Part print with two shaded views. Sizes in mm from the minimum x, y, z corner. A direction names the side the tool comes from. Coordinates: 2 decimals unless noted, no trailing zeros. Loops run counter-clockwise (first coordinate to the right, second up) from the corner with the lowest first, then second, coordinate; pieces in that order, holes last. Notation, with made-up numbers: (-34.5, -29) - (-0.5, -29) arc R22 ccw to (-0.5, 1) - close; hole circle Ø5 at (-4, 29.5). An arc over 180 degrees is marked (long way). Write each question's results on one line, items separated by ' | '. Start each with the question number.
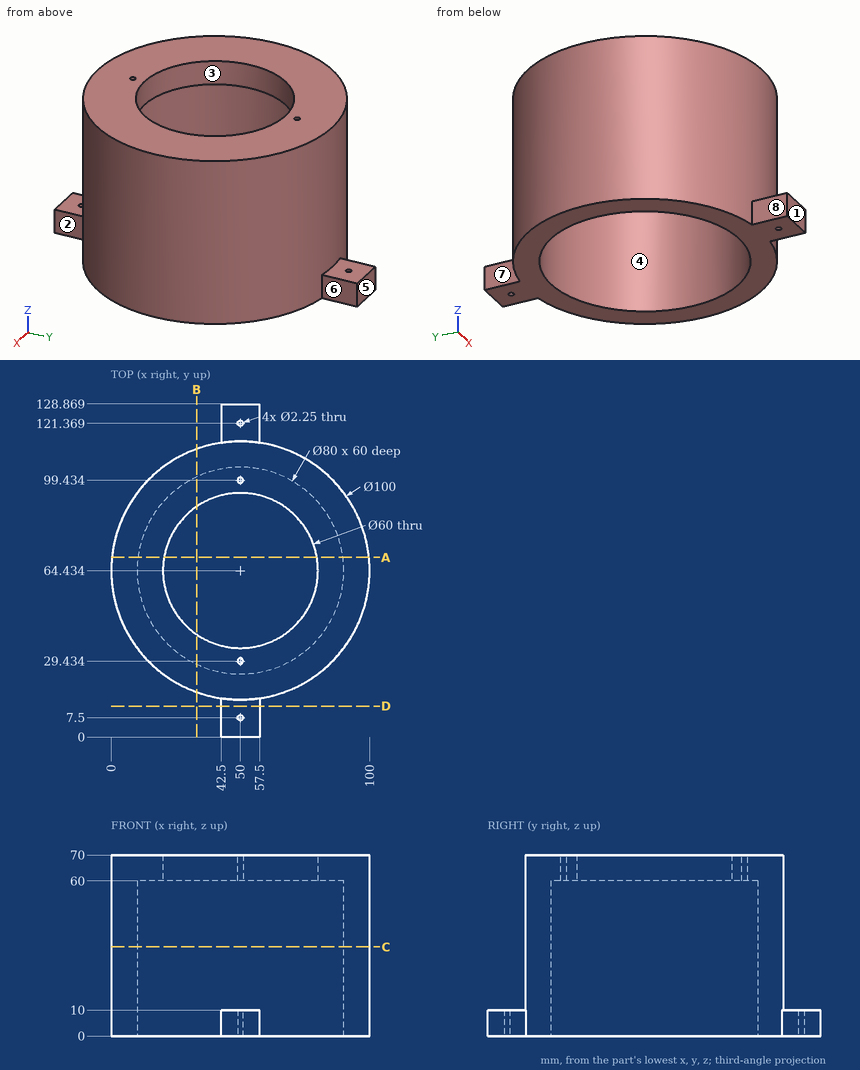
Q1. Pin check, flat tips, straight feed: pin 1 (12 mm diameter, centred on y = 53, z = 58.5, fed in from +X); pin 2 (4.5 mm diameter, centred on x = 53, y = 122.5, fed in from +Z); pin 3 (10 mm diameter, centred on x = 68, z = 17, fed in from +Y) (1 decimal). Stop position of each tip, or through.
Q2. Mould opens along Y. For the marked faces 1, 2 and 3 say: +Y half, -Y half, draft (parallel to the pull), parting line (faces both ways), or undercut.
Q3. Cut at A-A (y = 69.5). List the corners of the cut face in (x, z), and give its area (3 significant figures).
Q4. Cut at D-D (y = 12). List the corners of the cut face in (x, z), and give its area (3 significant figures).
Q5. Drill centre lines: L1, parallel to Y at x = 50, z = 62.5 (1 decimal); L2, parallel to Y at x = 48.5, z = 58; L3, parallel to Y at x = 50, z = 3.5 (1 decimal). Where is each one in solid material? Low to high. Write a range as from..to.
Q6. Which spindle directions (+Z, -Z, +X, -X, +Y, -Y) get a long thin tool onto all of the face, cutting with end or side? Do the marked faces 4, 5, 6, 7 and 8. Say none if no direction does.
Q7. Cut at C-C (z = 34.5). List the corners of the cut face in (x, y) (1 decimal), and give its area (3 significant figures).
Q8. Cut at B-B (x = 33). List the corners of the cut face in (y, z) (1 decimal).
Check result:
1) pin 1: x = 99.7 | pin 2: z = 10 | pin 3: y = 112.7
2) face 1: -Y half | face 2: draft | face 3: undercut
3) outline: (0.26, 0) - (10.32, 0) - (10.32, 60) - (20.43, 60) - (20.43, 70) - (0.26, 70) - close; (79.57, 60) - (89.68, 60) - (89.68, 0) - (99.74, 0) - (99.74, 70) - (79.57, 70) - close | area: 1,610 mm²
4) outline: (42.5, 0) - (57.5, 0) - (57.5, 10) - (42.5, 10) - close | area: 150 mm²
5) L1: 14.4..28.3, 30.6..34.4, 94.4..98.3, 100.6..114.4 | L2: 14.46..24.46, 104.41..114.41 | L3: 0..6.4, 8.6..24.4, 104.4..120.2, 122.5..128.9
6) face 4: -Z | face 5: +Z, -Z, +X, -X, +Y | face 6: +Z, -Z, +X, +Y | face 7: +Z, -Z, -X, +Y | face 8: +Z, -Z, -X, -Y
7) outline: circle Ø100 at (50, 64.4); hole circle Ø80 at (50, 64.4) | area: 2,830 mm²
8) outline: (17.4, 0) - (28.2, 0) - (28.2, 60) - (39.7, 60) - (39.7, 70) - (17.4, 70) - close; (89.2, 60) - (100.6, 60) - (100.6, 0) - (111.5, 0) - (111.5, 70) - (89.2, 70) - close
